from build123d import *

# Parameters (mm, degrees)
SKETCH1_W           = 150
SKETCH1_H           = 20
BOSS_EXTRUDE1_DEPTH = 10
FILLET1_R           = 10
SKETCH2_R           = 5
CUT_EXTRUDE1_DEPTH  = 152.657508881


with BuildPart() as part:
    # Sketch1 → Boss-Extrude1 (new body)
    with BuildSketch(Plane.XY):
        with Locations((75, 10)):
            Rectangle(SKETCH1_W, SKETCH1_H)
    extrude(amount=BOSS_EXTRUDE1_DEPTH)

    # Fillet1
    fillet1_edges = [part.edges().sort_by_distance(p)[0] for p in [
        (0, 0, 5),
        (150, 0, 5),
        (150, 20, 5),
        (0, 20, 5),
    ]]
    fillet(fillet1_edges, radius=FILLET1_R - 0.0001)  # a hair under: the kernel refuses the full size

    # Sketch2 → Cut-Extrude1 (cut, through all)
    with BuildSketch(Plane.XY.offset(10)):
        with Locations((10, 10)):
            Circle(SKETCH2_R)
        with Locations((140, 10)):
            Circle(SKETCH2_R)
    extrude(amount=-CUT_EXTRUDE1_DEPTH, mode=Mode.SUBTRACT)


solid = part.part
The model under review builds one solid part; all positions refer to its coordinate system, in mm. Round coordinates to 2 decimals unless told otherwise and drop trailing zeros. Write each loop counter-clockwise with the first axis right and the second up, starting at its lowest first coordinate (ties: lowest second). Pieces come first, ordered by that corner, then holes. Notation, with made-up numbers: (7.5, 82.5) - (21.5, 82.5) arc R3 cw to (21.5, 86.5) - close; hole circle Ø9 at (0, -28). An arc over 180 degrees is marked (long way). One line per item, written item: value. Start each with the question number.
1. Consider section A-A on z = 8. State how many separate pieces and enclosed holes the cut face has, and give its area (3 significant figures).
2. To check wall thickness, follow L1, parallel to X at y = 9.75, z = 1.5; L2, parallel to X at y = 12.75, z = 6; L3, parallel to Y at x = 10, z = 5. State the ranges of each line that lie inside material, in increasing order. Write a range as from..to.
3. The part is to be moulded in two halves that separate along Y. For faces 1 (the face through (147.15, 16.99, 5.07)), 2 (the face through (135, 10, 5)), 3 (the face through (2.85, 3.01, 5.07)), say which applies: released by +Y, released by -Y, zero draft, split by the parting line, or undercut.
4. Clearance check with flat-ended pins moving along their axes: P1, Ø3, axis at y = 7, z = 3, coming from the +X side; P2, Ø3, axis at y = 15.5, z = 8.5, coming from the -X side. State where each tip first meets the part, or that it passes through.
5. Consider section B-B on y = 7.25. Write out the cut boundary in (x, z).
Checks:
1. separate pieces: 1
1. enclosed holes: 2
1. area: 2,760 mm^2
2. L1: x = 0..5.01, 14.99..135.01, 144.99..150
2. L2: x = 0.39..5.82, 14.18..135.82, 144.18..149.61
2. L3: y = 0..5, 15..20
3. face 1: released by +Y
3. face 2: undercut
3. face 3: released by -Y
4. P1: stops at x = 149.89
4. P2: stops at x = 0.83
5. outline: (0.39, 0) - (5.82, 0) - (5.82, 10) - (0.39, 10) - close; (14.18, 0) - (135.82, 0) - (135.82, 10) - (14.18, 10) - close; (144.18, 0) - (149.61, 0) - (149.61, 10) - (144.18, 10) - close
